Model file for the job. Use its own axes, mm. Round coordinates to 2 decimals unless told otherwise and drop trailing zeros. Order: outer loops, then holes, each group sorted by start corner. A loop starts at its lowest first (then second) coordinate and runs counter-clockwise, first axis right, second up. Notation, with made-up numbers: (-27.5, 56.25) -> (3.5, 56.25) arc R25 cw to (3.5, 81.25) -> close; hole circle Ø1 at (-9, -32.75). An arc over 180 degrees is marked (long way). Use CSV: the item, a comma, the result in double quotes.
Autodesk Inventor part; units mm, degrees
ref_plane "YZ Plane" through (0, 0, 0) normal (1, 0, 0) x (0, 1, 0)
ref_plane "XZ Plane" through (0, 0, 0) normal (0, 1, 0) x (-1, 0, 0)
ref_plane "XY Plane" through (0, 0, 0) normal (0, 0, 1) x (1, 0, 0)
ref_plane "Work Plane1" through (0, 0, 0) normal (0, 0, 1) x (1, 0, 0)
ref_plane "Work Plane2" through (0, 0, 0) normal (0, 0, 1) x (1, 0, 0)
sketch "Sketch3" plane through (0, 0, 0) normal (0, 0, 1) x (1, 0, 0)
  circle A0 centre (3, -25.75) radius 2.3
  circle A1 centre (3, -3) radius 2.3
  circle A2 centre (3, -74.8889) radius 2.3
  line L0 (0, 0) -> (6, 0)
  line L1 (0, -77.8889) -> (0, 0)
  line L2 (0, -77.8889) -> (6, -77.8889)
  line L3 (6, -71.8889) -> (6, -77.8889)
  line L4 (6, -71.8889) -> (1.6, -71.8889)
  line L5 (1.6, -71.8889) -> (1.6, -56.7889)
  line L6 (1.6, -56.7889) -> (9.6, -56.7889)
  line L7 (9.6, -44.7889) -> (9.6, -56.7889)
  line L8 (3, -44.7889) -> (9.6, -44.7889)
  line L9 (3, -28.75) -> (3, -44.7889)
  line L10 (3, -28.75) -> (6, -28.75)
  line L11 (6, -28.75) -> (6, -22.75)
  line L12 (6, -22.75) -> (3, -22.75)
  line L13 (3, -6) -> (3, -22.75)
  line L14 (3, -6) -> (6, -6)
  line L15 (6, -6) -> (6, 0)
  circle A3 centre (5.6, -52.7889) radius 2.6
  circle A4 centre (175, -3) radius 2.3
  circle A5 centre (175, -25.75) radius 2.3
  line L16 (175, -28.75) -> (175, -41.8889)
  line L17 (168.4, -41.8889) -> (175, -41.8889)
  line L18 (168.4, -53.8889) -> (168.4, -41.8889)
  line L19 (175, -53.8889) -> (168.4, -53.8889)
  line L20 (175, -53.8889) -> (175, -71.8889)
  line L21 (172, -71.8889) -> (172, -77.8889)
  line L22 (178, -77.8889) -> (172, -77.8889)
  line L23 (178, -77.8889) -> (178, 0)
  line L24 (178, 0) -> (172, 0)
  line L25 (172, 0) -> (172, -6)
  line L26 (172, -6) -> (175, -6)
  line L27 (175, -6) -> (175, -22.75)
  line L28 (175, -22.75) -> (172, -22.75)
  line L29 (172, -22.75) -> (172, -28.75)
  line L30 (172, -28.75) -> (175, -28.75)
  circle A6 centre (175, -74.8889) radius 2.3
  circle A7 centre (172.4, -49.8889) radius 2.6
  circle A8 centre (89, 0.9661) radius 2.3
  circle A9 centre (89, 29.5) radius 2.3
  circle A10 centre (89, 15.55) radius 3.3
  circle A11 centre (89, -14.375) radius 3.3
  circle A12 centre (89, 41.2) radius 3.3
  line L31 (93.5, -27.75) -> (84.5, -27.75)
  line L32 (93.5, 55) -> (93.5, -27.75)
  line L33 (84.5, 55) -> (93.5, 55)
  line L34 (84.5, -27.75) -> (84.5, 55)
  line L35 (105.5, -27.75) -> (111.5, -27.75)
  line L36 (111.5, -24.9105) -> (111.5, -27.75)
  arc A13 (105.5, -24.9105) -> (111.5, -24.9105) centre (108.5, -23.95) ccw
  line L37 (105.5, -27.75) -> (105.5, -24.9105)
  arc A14 (111.5, -22.9895) -> (105.5, -22.9895) centre (108.5, -23.95) ccw
  line L38 (111.5, -5.5855) -> (111.5, -22.9895)
  arc A15 (105.5, -5.5855) -> (111.5, -5.5855) centre (108.5, -4.625) ccw
  line L39 (105.5, -22.9895) -> (105.5, -5.5855)
  circle A16 centre (108.4846, 4.5875) radius 2.3
  arc A17 (105.5, 12.8395) -> (111.5, 12.8395) centre (108.5, 13.8) ccw
  line L40 (105.5, -3.6645) -> (105.5, 12.8395)
  arc A18 (111.5, -3.6645) -> (105.5, -3.6645) centre (108.5, -4.625) ccw
  line L41 (111.5, 12.8395) -> (111.5, -3.6645)
  circle A19 centre (108.4462, 27.5) radius 2.3
  arc A20 (111.5, 14.7605) -> (105.5, 14.7605) centre (108.5, 13.8) ccw
  line L42 (111.5, 40.6331) -> (111.5, 14.7605)
  arc A21 (105.5, 40.1338) -> (111.5, 40.6331) centre (108.4231, 41.3077) ccw
  line L43 (105.5, 14.7605) -> (105.5, 40.1338)
  arc A22 (111.5, 41.9823) -> (105.5, 42.4816) centre (108.4231, 41.3077) ccw
  line L44 (111.5, 55) -> (111.5, 41.9823)
  line L45 (105.5, 55) -> (111.5, 55)
  line L46 (105.5, 42.4816) -> (105.5, 55)
  line L47 (111.5, 41.9823) -> (111.5, 55)
  line L48 (111.5, 41.9823) -> (112.5, 41.9823)
  line L49 (112.5, 41.9823) -> (112.5, 55)
  line L50 (111.5, 55) -> (112.5, 55)
  line L51 (111.5, 14.7605) -> (111.5, 40.6331)
  line L52 (111.5, 14.7605) -> (112.5, 14.7605)
  line L53 (112.5, 14.7605) -> (112.5, 40.6331)
  line L54 (111.5, 40.6331) -> (112.5, 40.6331)
  line L55 (111.5, -3.6645) -> (111.5, 12.8395)
  line L56 (111.5, -3.6645) -> (112.5, -3.6645)
  line L57 (112.5, -3.6645) -> (112.5, 12.8395)
  line L58 (111.5, 12.8395) -> (112.5, 12.8395)
  line L59 (66.5, 14.7605) -> (66.5, 40.6331)
  line L60 (66.5, 40.6331) -> (65.5, 40.6331)
  line L61 (65.5, 14.7605) -> (65.5, 40.6331)
  line L62 (66.5, 14.7605) -> (65.5, 14.7605)
  line L63 (66.5, 41.9823) -> (66.5, 55)
  line L64 (66.5, 55) -> (65.5, 55)
  line L65 (65.5, 41.9823) -> (65.5, 55)
  line L66 (66.5, 41.9823) -> (65.5, 41.9823)
  line L67 (66.5, -3.6645) -> (66.5, 12.8395)
  line L68 (66.5, 12.8395) -> (65.5, 12.8395)
  line L69 (65.5, -3.6645) -> (65.5, 12.8395)
  line L70 (66.5, -3.6645) -> (65.5, -3.6645)
  arc A23 (66.5, -5.5855) -> (72.5, -5.5855) centre (69.5, -4.625) ccw
  line L71 (66.5, -22.9895) -> (66.5, -5.5855)
  arc A24 (72.5, -22.9895) -> (66.5, -22.9895) centre (69.5, -23.95) ccw
  line L72 (72.5, -5.5855) -> (72.5, -22.9895)
  line L73 (66.5, -27.75) -> (72.5, -27.75)
  line L74 (72.5, -24.9105) -> (72.5, -27.75)
  arc A25 (66.5, -24.9105) -> (72.5, -24.9105) centre (69.5, -23.95) ccw
  line L75 (66.5, -27.75) -> (66.5, -24.9105)
  circle A26 centre (69.5, 4.5875) radius 2.3
  arc A27 (72.5, -3.6645) -> (66.5, -3.6645) centre (69.5, -4.625) ccw
  line L76 (72.5, 12.8395) -> (72.5, -3.6645)
  arc A28 (66.5, 12.8395) -> (72.5, 12.8395) centre (69.5, 13.8) ccw
  line L77 (66.5, -3.6645) -> (66.5, 12.8395)
  circle A29 centre (69.5, 27.5) radius 2.3
  arc A30 (66.5, 40.6331) -> (72.5, 40.1338) centre (69.5769, 41.3077) ccw
  line L78 (66.5, 14.7605) -> (66.5, 40.6331)
  arc A31 (72.5, 14.7605) -> (66.5, 14.7605) centre (69.5, 13.8) ccw
  line L79 (72.5, 40.1338) -> (72.5, 14.7605)
  arc A32 (72.5, 42.4816) -> (66.5, 41.9823) centre (69.5769, 41.3077) ccw
  line L80 (72.5, 55) -> (72.5, 42.4816)
  line L81 (66.5, 55) -> (72.5, 55)
  line L82 (66.5, 41.9823) -> (66.5, 55)
  circle A33 centre (59.3, -21.5445) radius 1.75
  circle A34 centre (59.3, -7.2055) radius 1.75
  line L83 (56.8, -28.75) -> (56.8, 0)
  line L84 (61.8, -28.75) -> (56.8, -28.75)
  line L85 (61.8, 0) -> (61.8, -28.75)
  line L86 (61.8, 0) -> (56.8, 0)
  circle A35 centre (64.05, -19.8657) radius 1.75
  circle A36 centre (64.05, -8.8843) radius 1.75
  line L87 (61.8, 0) -> (61.8, -28.75)
  line L88 (61.8, -28.75) -> (66.3, -28.75)
  line L89 (66.3, 0) -> (66.3, -28.75)
  line L90 (61.8, 0) -> (66.3, 0)
  circle A37 centre (113.95, -19.8657) radius 1.75
  circle A38 centre (113.95, -8.8843) radius 1.75
  line L91 (116.2, 0) -> (116.2, -28.75)
  line L92 (116.2, 0) -> (111.7, 0)
  line L93 (111.7, 0) -> (111.7, -28.75)
  line L94 (116.2, -28.75) -> (111.7, -28.75)
  circle A39 centre (118.7, -21.5445) radius 1.75
  circle A40 centre (118.7, -7.2055) radius 1.75
  line L95 (121.2, -28.75) -> (121.2, 0)
  line L96 (116.2, 0) -> (121.2, 0)
  line L97 (116.2, 0) -> (116.2, -28.75)
  line L98 (116.2, -28.75) -> (121.2, -28.75)
  line L99 (0, 0) -> (178, 0)
  line L100 (178, 0) -> (178, -28.75)
  line L101 (178, -28.75) -> (0, -28.75)
  line L102 (0, -28.75) -> (0, 0)
  line L103 (112.5, 0) -> (65.5, 0)
  line L104 (65.5, 0) -> (65.5, 55)
  line L105 (65.5, 55) -> (112.5, 55)
  line L106 (112.5, 55) -> (112.5, 0)
  line L107 (104.5, 11.4325) -> (104.5, -10.5675)
  line L108 (94.5, -10.5675) -> (94.5, 11.4325)
  line L109 (104.5, 11.4325) -> (73.5, 11.4325)
  line L110 (73.5, 11.4325) -> (73.5, -10.5675)
  line L111 (73.5, -10.5675) -> (104.5, -10.5675)
  line L112 (104.5, -10.5675) -> (104.5, 11.4325)
  line L113 (72.5, 12.4325) -> (105.5, 12.4325)
  line L114 (105.5, 12.4325) -> (105.5, -11.5675)
  line L115 (105.5, -11.5675) -> (72.5, -11.5675)
  line L116 (72.5, -11.5675) -> (72.5, 12.4325)
  line L117 (175, -71.8889) -> (172, -71.8889)
  point P0 (112.5, 0)
  point P1 (65.5, 0)
  point P2 (0, -28.75)
  point P3 (172, 0)
  point P4 (93.5, 12.4325)
  point P5 (105.5, -5.5855)
  point P6 (93.5, -11.5675)
  point P7 (84.5, -11.5675)
  point P8 (72.5, -5.5855)
  point P9 (84.5, 12.4325)
  dimension "d29" = 1
  dimension "d30" = 1
  dimension "d31" = 1
extrude "Extrusion2" add sketch "Sketch3" along normal blind 2 contours A0 | A1 | L0 L15 L14 L13 L12 L11 L10 L101 L1 | L99 L83 L101 L11 L12 L13 L14 L15 | L86 L85 L84 L83 | L90 L69 L70 L89 L88 L85 | L90 L89 L70 L69 | L69 L68 L67 L99 L90 | L89 L70 A27 L116 A23 L71 A24 L72 L115 L34 L31 L32 L39 A14 L38 A15 L114 A18 L56 L93 L101 | L104 L62 A31 L79 A30 L60 L66 A32 L80 L105 L34 L113 L76 A28 L68 | L99 L67 L70 L89 | L93 L56 L57 L92 L91 L94 | A28 L76 L99 L67 | L61 L60 L59 L62 | L99 L76 A27 L67 | L93 L92 L57 L56 | L56 L41 L99 L93 | L91 L96 L95 L98 | L59 A30 L79 A31 | A18 L40 L99 L41 | L99 L41 L58 L57 L92 | L95 L99 L25 L26 L27 L28 L29 L101 | L65 L64 L63 L66 | L72 A24 L71 A23 | L99 L40 A17 L41 | L29 L28 L27 L26 L25 L24 L23 L101 L30 | L113 A10 L32 L109 L34 | L34 L33 L32 L113 A10 | L63 L81 L80 A32 | L99 A8 L32 L111 L34 | L34 L109 L32 L99 A8 | A15 L38 A14 L39 | A17 L40 L113 L32 L105 L46 A22 L48 L106 L54 A21 L43 A20 L52 L58 | L113 A10 | A10 L113 | L111 L32 L115 A11 L34 | L99 A8 | A8 L99 | L115 A11 L32 L31 L34 | L52 L42 L54 L53 | L115 A11 | A11 L115 | A20 L43 A21 L42 | L45 L44 A22 L46 | L48 L44 L50 L49 | A4 | A5 | A9 | A12 | L37 A13 L36 L35 | A16 | A19 | L75 A25 L74 L73 | A26 | A29 | A33 | A34 | A35 | A36 | A37 | A38 | A39 | A40
sketch "Sketch4" plane through (0, 0, 2) normal (0, 0, 1) x (1, 0, 0)
  circle A0 centre (69.5, 27.5) radius 2.3
  circle A1 centre (69.5, 4.5875) radius 2.3
  circle A2 centre (89, 0.9661) radius 2
  circle A3 centre (89, 29.5) radius 2.3
  circle A4 centre (108.4462, 27.5) radius 2.3
  circle A5 centre (108.4846, 4.5875) radius 2.3
  circle A6 centre (64.05, -8.8843) radius 1.75
  circle A7 centre (59.3, -7.2055) radius 1.75
  circle A8 centre (59.3, -21.5445) radius 1.75
  circle A9 centre (64.05, -19.8657) radius 1.75
  circle A10 centre (118.7, -21.5445) radius 1.75
  circle A11 centre (113.95, -19.8657) radius 1.75
  circle A12 centre (113.95, -8.8843) radius 1.75
  circle A13 centre (118.7, -7.2055) radius 1.75
  circle A14 centre (3, -25.75) radius 2.3
  circle A15 centre (3, -3) radius 2.3
  circle A16 centre (175, -25.75) radius 2.3
  circle A17 centre (175, -3) radius 2.3
  point P0 (0, 0)
hole "Hole2" at (3, -3, 2) at (3, -25.75, 2) at (175, -3, 2) at (175, -25.75, 2) at (108.4846, 4.5875, 2) at (89, 0.9661, 2) at (69.5, 4.5875, 2) at (69.5, 27.5, 2) at (89, 29.5, 2) at (108.4462, 27.5, 2) direction (0, 0, -1) diameter 3.6 end through all countersink diameter 6 countersink angle 90
sketch "Sketch5" plane through (0, 0, 2) normal (0, 0, 1) x (1, 0, 0)
  circle A0 centre (64.05, -19.8657) radius 1.75
  circle A1 centre (59.3, -21.5445) radius 1.75
  circle A2 centre (59.3, -7.2055) radius 1.75
  circle A3 centre (64.05, -8.8843) radius 1.75
  circle A4 centre (113.95, -8.8843) radius 1.75
  circle A5 centre (118.7, -7.2055) radius 1.75
  circle A6 centre (118.7, -21.5445) radius 1.75
  circle A7 centre (113.95, -19.8657) radius 1.75
  point P0 (0, 0)
hole "Hole3" at (59.3, -7.2055, 2) at (64.05, -8.8843, 2) at (64.05, -19.8657, 2) at (59.3, -21.5445, 2) at (113.95, -8.8843, 2) at (118.7, -7.2055, 2) at (118.7, -21.5445, 2) at (113.95, -19.8657, 2) direction (0, 0, -1) diameter 3.1 end through all countersink diameter 5 countersink angle 90
equation "\"d30\" = d29"
properties part number "ceil"
Q1. Cut at A-A (x = 102.5). Give the cut face in (y, z).
From the geometry:
outline,"(-28.75, 0) -> (-11.57, 0) -> (-11.57, 2) -> (-28.75, 2) -> close; (12.43, 0) -> (55, 0) -> (55, 2) -> (12.43, 2) -> close"
Q2. Cut at B-B (z = 0.3). State how many separate pieces and enclosed holes the cut face has, plus the area to 3 significant figures.
From the geometry:
separate pieces,"1"
enclosed holes,"20"
area,"6,960 mm²"
Q3. Probe line 1 along X through (y, z) = (-3, 0.2); line 2 along Y through (x, z) = (175, 0.5); line 3 along X through (y, z) = (10.5, 0.4). List the from-to ranges inside material, lowest first.
From the geometry:
line 1,"x = 0 to 1.2, 4.8 to 72.5, 84.5 to 93.5, 105.5 to 173.2, 176.8 to 178"
line 2,"y = -28.75 to -27.55, -23.95 to -4.8, -1.2 to 0"
line 3,"x = 65.5 to 72.5, 84.5 to 93.5, 105.5 to 112.5"
Q4. Pin check, flat tips, straight feed: pin 1 (4 mm diameter, centred on x = 3, y = -3, fed in from +Z); pin 2 (4.5 mm diameter, centred on x = 108.48, y = 4.59, fed in from +Z); pin 3 (1 mm diameter, centred on y = 1.5, z = 1, fed in from +X). Stop position of each tip, or through.
From the geometry:
pin 1,"stops at z = 1"
pin 2,"stops at z = 1.26"
pin 3,"stops at x = 112.5"
Q5. Mould opens along Y. For faces 1 (the conical face through (87, 1, 1)), 2 (the flat face through (177.3, -0.6, 2)) say: +Y half, -Y half, draft (parallel to the pull), parting line (faces both ways), or undercut.
From the geometry:
face 1,"undercut"
face 2,"draft"
Q6. Cut at D-D (x = 28.5). Give the cut face in (y, z), plus the area to 3 significant figures.
From the geometry:
outline,"(-28.75, 0) -> (0, 0) -> (0, 2) -> (-28.75, 2) -> close"
area,"57.5 mm²"
Q7. Cut at C-C (y = 22). Give the cut face in (x, z).
From the geometry:
outline,"(65.5, 0) -> (112.5, 0) -> (112.5, 2) -> (65.5, 2) -> close"
